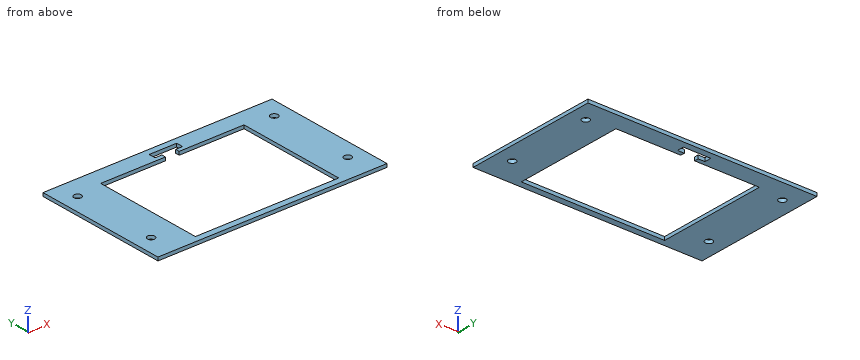
from build123d import *

# Parameters (mm, degrees)
SKETCH1_W             = 107.95
SKETCH1_H             = 63.5
BOSS_EXTRUDE1_DEPTH   = 1.5875
SKETCH2_W             = 67.564
SKETCH2_H             = 52.324
CUT_EXTRUDE1_DEPTH    = 63.640907411
F_4_CLEARANCE_HOLE1_D = 3.4544


with BuildPart() as part:
    # Sketch1 → Boss-Extrude1 (new body)
    with BuildSketch(Plane.XY):
        Rectangle(SKETCH1_W, SKETCH1_H)
    extrude(amount=BOSS_EXTRUDE1_DEPTH)

    # Sketch2 → Cut-Extrude1 (cut, through all)
    with BuildSketch(Plane.XY.offset(1.5875)):
        with Locations((0, -2.6035)):
            Rectangle(SKETCH2_W, SKETCH2_H)
        Polygon((-3.2385, 25.527), (-3.2385, 23.5585), (3.2385, 23.5585), (3.2385, 25.527), (6.477, 25.527), (6.477, 28.7655), (-6.477, 28.7655), (-6.477, 25.527), align=None)
    extrude(amount=-CUT_EXTRUDE1_DEPTH, mode=Mode.SUBTRACT)

    # 4 Clearance Hole1 (through all)
    with Locations(Plane.XY.offset(1.5875)):
        with Locations((-46.355, 21.59), (-46.355, -19.05), (46.355, 21.59), (46.355, -19.05)):
            Hole(F_4_CLEARANCE_HOLE1_D / 2)


solid = part.part
Model file for the job. Use its own axes, mm. Coordinates: 2 decimals unless noted, no trailing zeros. Order: outer loops, then holes, each group sorted by start corner. A loop starts at its lowest first (then second) coordinate and runs counter-clockwise, first axis right, second up. Notation, with made-up numbers: (-29.5, 74) -> (-8.5, 74) arc R37 cw to (-8.5, 110) -> close; hole circle Ø7 at (6, 20). An arc over 180 degrees is marked (long way). Return JSON: item names as keys, results as strings. Group by question number.
Item 1: Saw through at C-C on z = 1.2. State how many separate pieces and enclosed holes the cut face has, then the cut area to 3 significant figures.
Item 2: Wall check: line 1 along Y through (x, z) = (-7.5, 1.55); line 2 along Y through (x, z) = (-4, 1.55); line 3 along X through (y, z) = (13.5, 0.2) (3 decimals). Give the ranges that are in metal, low to high. Write a range as [from, to].
Item 3: Flat gauge pin, fed straight in: P1, Ø2, axis at x = -46.355, y = -19.05, coming from the -Z side. Where does the tip first touch, or does it go through?
Item 4: Saw through at B-B on x = 26.5. Write the cut outline in (y, z), then the cut area to 3 significant figures.
Item 5: Saw through at A-A on y = -19.05. Write the cut outline in (x, z) (1 decimal), then the cut area to 3 significant figures.
Values found:
{
 "1": {"separate pieces": "1", "enclosed holes": "5", "area": "3,230 mm2"},
 "2": {"line 1": "y = [-31.75, -28.77], [23.56, 31.75]", "line 2": "y = [-31.75, -28.77], [23.56, 25.53], [28.77, 31.75]", "line 3": "x = [-53.975, -33.782], [33.782, 53.975]"},
 "3": {"P1": "passes through"},
 "4": {"outline": "(-31.75, 0) -> (-28.77, 0) -> (-28.77, 1.59) -> (-31.75, 1.59) -> close; (23.56, 0) -> (31.75, 0) -> (31.75, 1.59) -> (23.56, 1.59) -> close", "area": "17.7 mm2"},
 "5": {"outline": "(-54, 0) -> (-48.1, 0) -> (-48.1, 1.6) -> (-54, 1.6) -> close; (-44.6, 0) -> (-33.8, 0) -> (-33.8, 1.6) -> (-44.6, 1.6) -> close; (33.8, 0) -> (44.6, 0) -> (44.6, 1.6) -> (33.8, 1.6) -> close; (48.1, 0) -> (54, 0) -> (54, 1.6) -> (48.1, 1.6) -> close", "area": "53.1 mm2"}
}
